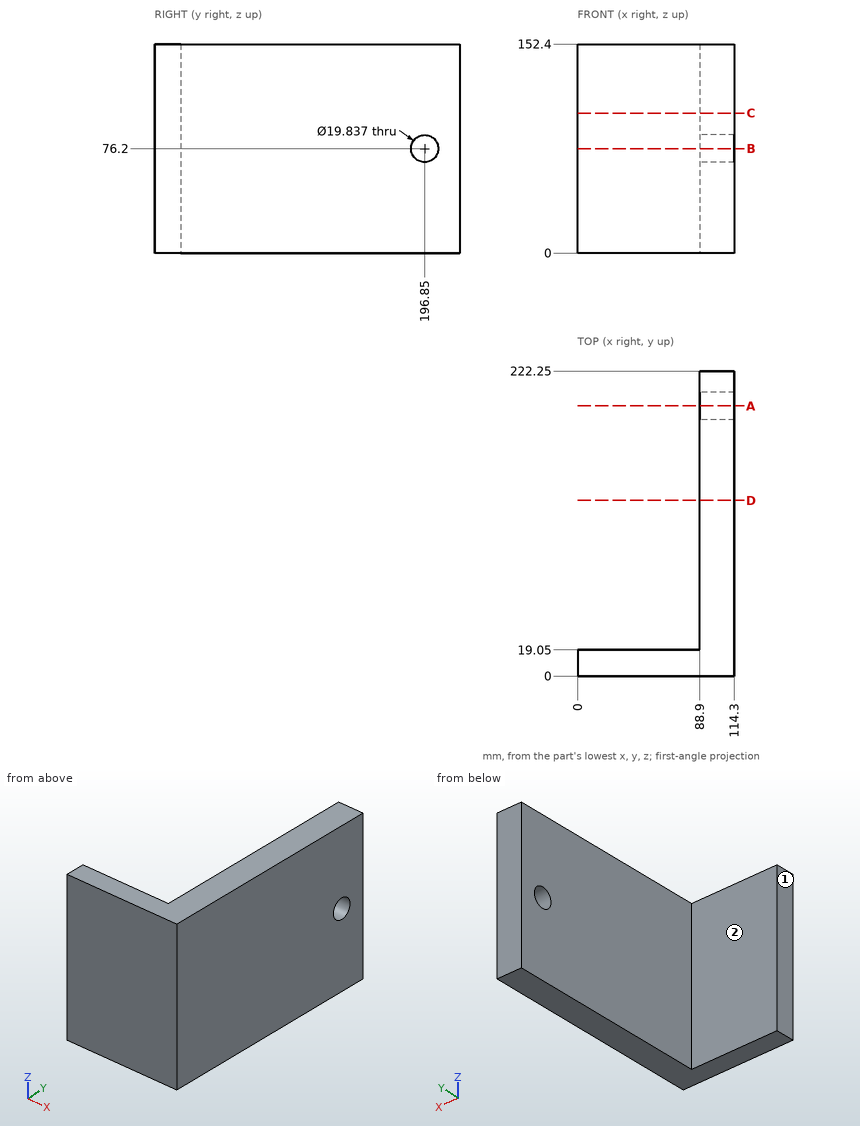
Geometry check sheet. Reference: drawing and pictorial views, mm from the part's lowest x, y, z. A direction names the side the tool comes from. Round coordinates to 2 decimals unless told otherwise and drop trailing zeros. Order: outer loops, then holes, each group sorted by start corner. A loop starts at its lowest first (then second) coordinate and runs counter-clockwise, first axis right, second up.
Q1. Cross-section at C-C, the plane z = 102. Enter the section's corners in (x, y).
Filled sheet:
outline: (0, 0) - (114.3, 0) - (114.3, 222.25) - (88.9, 222.25) - (88.9, 19.05) - (0, 19.05) - close
Q2. Depth check by flat-ended pin: P1, Ø10, axis at x = 73, z = 19.5, coming from the +Y side. Enter the tip coordinate at first touch or a pass-through.
Filled sheet:
P1: stops at y = 19.05
Q3. Cross-section at D-D, the plane y = 128. Enter the section's corners in (x, z), plus the area to 3 significant figures.
Filled sheet:
outline: (88.9, 0) - (114.3, 0) - (114.3, 152.4) - (88.9, 152.4) - close
area: 3,870 mm2
Q4. Cross-section at B-B, the plane z = 76.2. Enter the section's corners in (x, y).
Filled sheet:
outline: (0, 0) - (114.3, 0) - (114.3, 186.93) - (88.9, 186.93) - (88.9, 19.05) - (0, 19.05) - close; (88.9, 206.77) - (114.3, 206.77) - (114.3, 222.25) - (88.9, 222.25) - close
Q5. Set-up check for the marked faces 1 and 2: record each of +Z, -Z, +X, -X, +Y, -Y from which the full face is reachable in a straight line by a thin tool's end or side.
Filled sheet:
face 1: +Z, -Z, -X, +Y, -Y
face 2: +Z, -Z, -X, +Y
Q6. Scan lines: L1, parallel to Z at x = 94, y = 196; L2, parallel to Y at x = 105.75, z = 76.2; L3, parallel to Y at x = 69, z = 121. Record each from-to range of solid material in increasing order.
Filled sheet:
L1: z = 0 to 66.32, 86.08 to 152.4
L2: y = 0 to 186.93, 206.77 to 222.25
L3: y = 0 to 19.05
Q7. Cross-section at A-A, the plane y = 196.85. Enter the section's corners in (x, z).
Filled sheet:
outline: (88.9, 0) - (114.3, 0) - (114.3, 66.28) - (88.9, 66.28) - close; (88.9, 86.12) - (114.3, 86.12) - (114.3, 152.4) - (88.9, 152.4) - close
